Source: three-view drawing plus pictorial views. Frame: mm from the lowest corner of the part. A direction names the side the tool comes from. Round coordinates to 2 decimals unless told otherwise and drop trailing zeros. Loops run counter-clockwise (first coordinate to the right, second up) from the corner with the lowest first, then second, coordinate; pieces in that order, holes last. Notation, with made-up numbers: (-9.75, 14) -> (46.25, 14) arc R9 cw to (46.25, 21) -> close; hole circle Ø4 at (-34.75, 89). An arc over 180 degrees is marked (long way). Return JSON: item names as keys, results as strings. Group by question number.
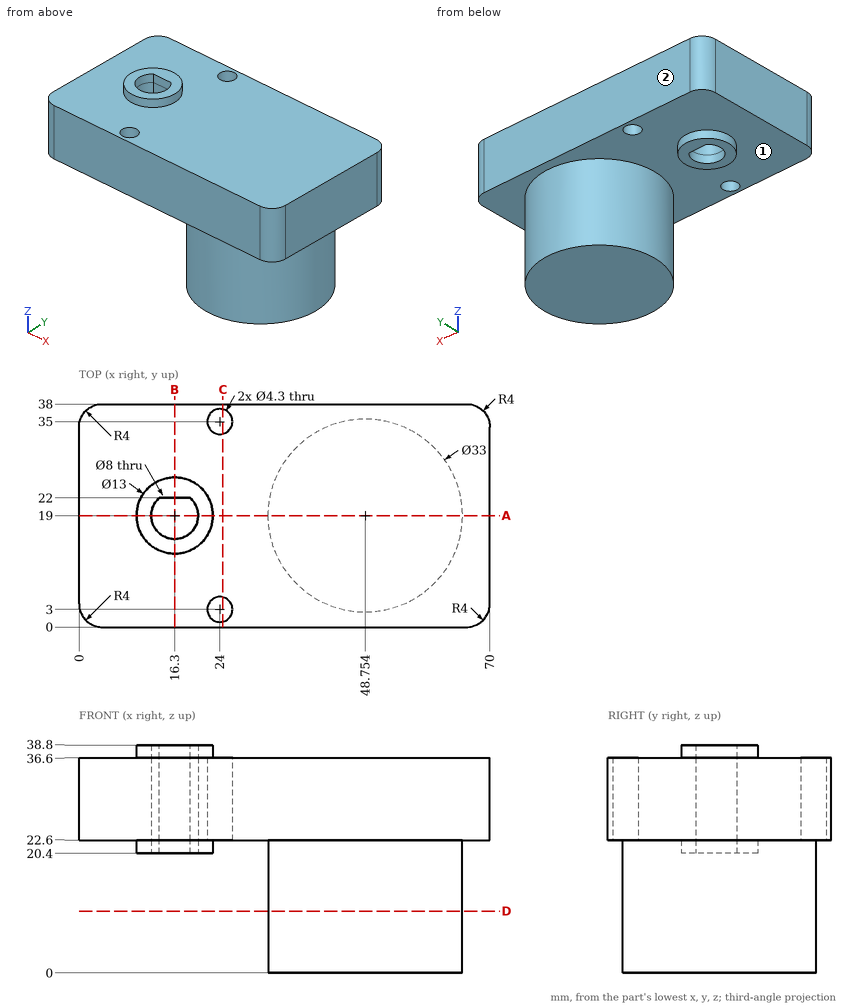
(1) Ray query, line 1 (Y direction, x = 16, z = 37); line 2 (X direction, y = 19, z = 26); line 3 (Z direction, x = 31, y = 13.5). Return the intervals inside material, ascending.
(2) Set-up query: the marked faces 1 and 2. Return all of +Z, -Z, +X, -X, +Y, -Y with unobstructed straight access to the full face (end or side cutting, diameter ignored); none if empty.
(3) Cut plane C-C (x = 24.5). Return loops of the section in (y, z).
(4) Cut plane B-B (x = 16.3). Return loops of the section in (y, z), and give its area (3 significant figures).
(5) Cut plane A-A (y = 19). Return loops of the section in (x, z), and give its area (3 significant figures).
(6) Pin query (flat end, axial travel): pin 1 (9 mm diameter, centred on x = 16.3, y = 19, fed in from -Z); pin 2 (0.7 mm diameter, centred on x = 15.5, z = 22, fed in from -Y); pin 3 (5.5 mm diameter, centred on x = 24, y = 35, fed in from +Z). Return the tip coordinate at first contact, or that it passes through.
(7) Cut plane D-D (z = 10.5). Return loops of the section in (x, y).
Answers follow:
{
 "1": {"line 1": "12.51 to 15.01, 22 to 25.49", "line 2": "0 to 12.3, 20.3 to 70", "line 3": "22.6 to 36.6"},
 "2": {"face 1": "-Z", "face 2": "+Z, -Z, +X, -X, +Y"},
 "3": {"outline": "(0, 22.6) -> (0.91, 22.6) -> (0.91, 36.6) -> (0, 36.6) -> close; (5.09, 22.6) -> (32.91, 22.6) -> (32.91, 36.6) -> (5.09, 36.6) -> close; (37.09, 22.6) -> (38, 22.6) -> (38, 36.6) -> (37.09, 36.6) -> close"},
 "4": {"outline": "(0, 22.6) -> (12.5, 22.6) -> (12.5, 20.4) -> (15, 20.4) -> (15, 38.8) -> (12.5, 38.8) -> (12.5, 36.6) -> (0, 36.6) -> close; (22, 20.4) -> (25.5, 20.4) -> (25.5, 22.6) -> (38, 22.6) -> (38, 36.6) -> (25.5, 36.6) -> (25.5, 38.8) -> (22, 38.8) -> close", "area": "460 mm^2"},
 "5": {"outline": "(0, 22.6) -> (9.8, 22.6) -> (9.8, 20.4) -> (12.3, 20.4) -> (12.3, 38.8) -> (9.8, 38.8) -> (9.8, 36.6) -> (0, 36.6) -> close; (20.3, 20.4) -> (22.8, 20.4) -> (22.8, 22.6) -> (32.25, 22.6) -> (32.25, 0) -> (65.25, 0) -> (65.25, 22.6) -> (70, 22.6) -> (70, 36.6) -> (22.8, 36.6) -> (22.8, 38.8) -> (20.3, 38.8) -> close", "area": "1,640 mm^2"},
 "6": {"pin 1": "z = 20.4", "pin 2": "y = 12.52", "pin 3": "z = 36.6"},
 "7": {"outline": "circle Ø33 at (48.75, 19)"}
}
